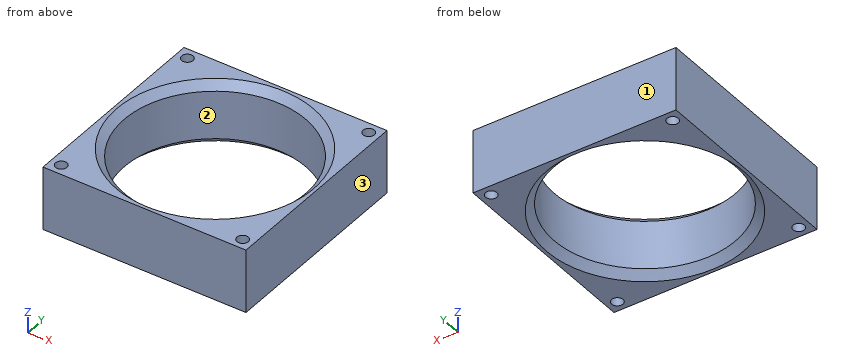
Autodesk Inventor part; units mm, degrees
ref_plane "YZ Plane" through (0, 0, 0) normal (1, 0, 0) x (0, 1, 0)
ref_plane "XZ Plane" through (0, 0, 0) normal (0, 1, 0) x (-1, 0, 0)
ref_plane "XY Plane" through (0, 0, 0) normal (0, 0, 1) x (1, 0, 0)
sketch "Sketch1" plane through (0, 0, 0) normal (0, 0, 1) x (1, 0, 0)
  line L0 (-40, -40) -> (40, -40)
  line L1 (40, -40) -> (40, 40)
  line L2 (40, 40) -> (-40, 40)
  line L3 (-40, 40) -> (-40, -40)
  point P0 (0, 0)
  point P1 (40, 0)
  point P2 (0, 40)
  dimension "L" = 80
  dimension "d1" = 80
extrude "Extrusion1" add sketch "Sketch1" along normal blind 25
sketch "Sketch2" plane through (0, 0, 25) normal (0, 0, 1) x (1, 0, 0)
  line L0 (-35.75, -35.75) -> (35.75, -35.75) construction
  line L1 (35.75, -35.75) -> (35.75, 35.75) construction
  line L2 (35.75, 35.75) -> (-35.75, 35.75) construction
  line L3 (-35.75, 35.75) -> (-35.75, -35.75) construction
  point P0 (0, 0)
  point P1 (-35.75, 0)
  point P2 (0, 35.75)
  dimension "inner" = 71.5
  dimension "d5" = 71.5
hole "Hole1" at (-35.75, 35.75, 25) at (35.75, 35.75, 25) at (-35.75, -35.75, 25) at (35.75, -35.75, 25) direction (0, 0, -1) diameter 4.5 end through all
sketch "Sketch3" plane through (0, 0, 25) normal (0, 0, 1) x (1, 0, 0)
  point P0 (0, 0)
  point P1 (0, 0)
hole "Hole2" at (0, 0, 25) direction (0, 0, -1) diameter 71.5 end through all
chamfer "Chamfer1" distance 3 angle 45 2 edges at (0, 35.75, 25) (0, 35.75, 0)
equation "\"d1\" = L"
equation "\"d5\" = inner"
properties part number "fan" material "ABS Plastic"
Design review of the part built by this model. Coordinates are the model's own, in mm. Face numbers are marked on the shaded views. Give positions to 0.01 mm unless a question says otherwise; leave off trailing zeros. Order: outer loops, then holes, each group sorted by start corner. A loop starts at its lowest first (then second) coordinate and runs counter-clockwise, first axis right, second up. Notation, with made-up numbers: (75.5, 18.25) - (99.5, 18.25) arc R21 ccw to (99.5, 56.25) - close; hole circle Ø2 at (-29.75, 55.25). An arc over 180 degrees is marked (long way). Use CSV: the item, a comma, the result in double quotes. Start each with the question number.
Q1. For line 1 (X direction, y = -12.5, z = 3.5); line 2 (Y direction, x = 0, z = 9.5); line 3 (X direction, y = -26.5, z = 3.5), list the stretches that pass through material, from the lowest coordinate up.
Q2. For P1, Ø4, axis at x = 35.75, y = 35.75, coming from the +Z side; P2, Ø12, axis at x = 31, y = 21, coming from the -Z side, all flat-tipped, find the tip position at first contact; note any pin that passes through.
Q3. Take a section at A-A (z = 23.5). State the section outline as (x, y) points, and give its area (3 significant figures).
Q4. Take a section at D-D (z = 15.75). State the section outline as (x, y) points, and give its area (3 significant figures).
Q5. Take a section at B-B (x = 0). State the section outline as (y, z) points.
Q6. Draft analysis for pull direction Y (two halves, no side actions). For the marked faces 1, 2 and 3, state which applies: pulls with the +Y half, pulls with the -Y half, needs draft (parallel to the pull), parting line crosses it, or undercut.
Calculated:
1,line 1,"x = -40 to -33.49, 33.49 to 40"
1,line 2,"y = -40 to -35.75, 35.75 to 40"
1,line 3,"x = -40 to -24, 24 to 40"
2,P1,"passes through"
2,P2,"stops at z = 0"
3,outline,"(-40, -40) - (40, -40) - (40, 40) - (-40, 40) - close; hole circle Ø4.5 at (-35.75, -35.75); hole circle Ø4.5 at (-35.75, 35.75); hole circle Ø74.5 at (0, 0); hole circle Ø4.5 at (35.75, -35.75); hole circle Ø4.5 at (35.75, 35.75)"
3,area,"1,980 mm²"
4,outline,"(-40, -40) - (40, -40) - (40, 40) - (-40, 40) - close; hole circle Ø4.5 at (-35.75, -35.75); hole circle Ø4.5 at (-35.75, 35.75); hole circle Ø71.5 at (0, 0); hole circle Ø4.5 at (35.75, -35.75); hole circle Ø4.5 at (35.75, 35.75)"
4,area,"2,320 mm²"
5,outline,"(-40, 0) - (-38.75, 0) - (-35.75, 3) - (-35.75, 22) - (-38.75, 25) - (-40, 25) - close; (35.75, 3) - (38.75, 0) - (40, 0) - (40, 25) - (38.75, 25) - (35.75, 22) - close"
6,face 1,"pulls with the +Y half"
6,face 2,"undercut"
6,face 3,"needs draft"
